Autodesk Inventor part; units mm, degrees
ref_plane "YZ Plane" through (0, 0, 0) normal (1, 0, 0) x (0, 1, 0)
ref_plane "XZ Plane" through (0, 0, 0) normal (0, 1, 0) x (-1, 0, 0)
ref_plane "XY Plane" through (0, 0, 0) normal (0, 0, 1) x (1, 0, 0)
sketch "Skizze1" plane through (0, 0, 0) normal (0, 0, 1) x (1, 0, 0)
  line L0 (0, 0) -> (10, 0)
  line L1 (10, 0) -> (10, 10)
  line L2 (10, 10) -> (0, 10)
  line L3 (0, 10) -> (0, 0)
  line L4 (70, 10) -> (80, 10)
  line L5 (80, 10) -> (80, 0)
  line L6 (80, 0) -> (70, 0)
  line L7 (70, 0) -> (70, 10)
  dimension "d0" = 10
  dimension "d1" = 10
  dimension "d2" = 10
  dimension "d3" = 10
  dimension "d4" = 60
extrude "Extrusion1" add sketch "Skizze1" along normal blind 7.5
sketch "Skizze2" plane through (0, 0, 7.5) normal (0, 0, 1) x (1, 0, 0)
  line L0 (80, 10) -> (70, 10)
  line L1 (70, 10) -> (70, 0)
  line L2 (70, 0) -> (80, 0)
  line L3 (80, 0) -> (80, 10)
  line L4 (0, 10) -> (80, 10)
  line L5 (80, 10) -> (80, 0)
  line L6 (80, 0) -> (0, 0)
  line L7 (0, 0) -> (0, 10)
extrude "Extrusion2" add sketch "Skizze2" along normal blind 4
fillet "Rundung1" radius 3 1 edges at (0, 5, 11.5)
fillet "Rundung1" radius 3 1 edges at (80, 5, 11.5)
fillet "Rundung1" radius 3 1 edges at (70, 5, 7.5)
fillet "Rundung1" radius 3 1 edges at (10, 5, 7.5)
sketch "Skizze3" plane through (0, 0, 7.5) normal (0, 0, -1) x (-1, 0, 0)
  line L0 (0, 0) -> (-50, 0)
  line L1 (-50, 0) -> (-50, 2)
  line L2 (-50, 2) -> (0, 2)
  line L3 (0, 2) -> (0, 0)
  dimension "d13" = 50
  dimension "d14" = 2
extrude "Extrusion3" add sketch "Skizze3" along normal blind 2
fillet "Rundung2" radius 1 1 edges at (50, 1, 5.5)
sketch "Skizze4" plane through (0, 0, 0) normal (0, 0, -1) x (-1, 0, 0)
  line L0 (0, 0) -> (-10, 0)
  line L1 (0, 10) -> (0, 0)
  circle A0 centre (-5, 5) radius 2.5
  dimension "d18" = 5
  dimension "d19" = 5
  dimension "d20" = 5
sketch "Skizze5" plane through (0, 0, 0) normal (0, 0, -1) x (-1, 0, 0)
  line L0 (-80, 0) -> (-70, 0)
  line L1 (-70, 0) -> (-70, 10)
  circle A0 centre (-75, 5) radius 2.5
  point P0 (0, 0)
  dimension "d21" = 5
  dimension "d22" = 5
  dimension "d23" = 5
extrude "Extrusion4" add sketch "Skizze4" along normal blind 3
extrude "Extrusion5" add sketch "Skizze5" along normal blind 3
properties part number "USB-Halter"
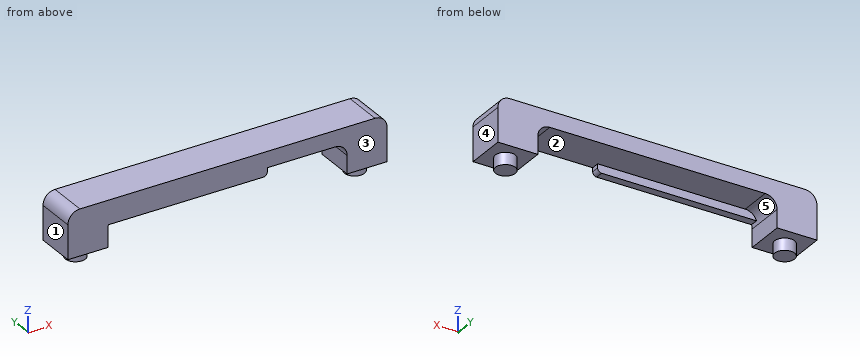
CAD build for the part. Positions are in the model's coordinates, mm. Face numbers are marked on the shaded views. A direction names the side the tool comes from. Give positions to 0.01 mm unless a question says otherwise; leave off trailing zeros. Loops run counter-clockwise (first coordinate to the right, second up) from the corner with the lowest first, then second, coordinate; pieces in that order, holes last. Notation, with made-up numbers: (15.5, 47) - (42.5, 47) arc R20 ccw to (42.5, 51) - close; hole circle Ø2 at (26.25, 8). An arc over 180 degrees is marked (long way). Put each result on its own line as item: value.
Q1. Slice it at C-C (y = 6). Give the cut face in (x, z).
Filled in:
outline: (0, 0) - (2.71, 0) - (2.71, -3) - (7.29, -3) - (7.29, 0) - (10, 0) - (10, 4.5) arc R3 cw to (13, 7.5) - (67, 7.5) arc R3 cw to (70, 4.5) - (70, 0) - (72.71, 0) - (72.71, -3) - (77.29, -3) - (77.29, 0) - (80, 0) - (80, 8.5) arc R3 ccw to (77, 11.5) - (3, 11.5) arc R3 ccw to (0, 8.5) - close
Q2. Mould opens along X. For the marked faces 1, 2 and 3 say: pulls with the +X half, pulls with the -X half, needs draft (parallel to the pull), parting line crosses it, or undercut.
Filled in:
face 1: pulls with the -X half
face 2: undercut
face 3: needs draft
Q3. Slice it at B-B (x = 75). Give the cut face in (y, z), plus the area to 3 significant figures.
Filled in:
outline: (0, 0) - (2.5, 0) - (2.5, -3) - (7.5, -3) - (7.5, 0) - (10, 0) - (10, 11.5) - (0, 11.5) - close
area: 130 mm²
Q4. Flat gauge pins, fed straight in: pin 1 (1.6 mm diameter, centred on x = 38, y = 0.5, fed in from -Z); pin 2 (2 mm diameter, centred on x = 37.5, z = 6, fed in from +Y). Where does each tip first touch, or does it go through?
Filled in:
pin 1: stops at z = 5.5
pin 2: stops at y = 2
Q5. Probe line 1 along X through (y, z) = (2.25, 4.75); line 2 along Z through (x, y) = (39, 1.25); line 3 along X through (y, z) = (4, 5.75). List the from-to ranges inside material, lowest first.
Filled in:
line 1: x = 0 to 10.01, 69.99 to 80
line 2: z = 5.5 to 11.5
line 3: x = 0 to 10.27, 69.73 to 80
Q6. Slice it at A-A (z = 3.75). Give the cut face in (x, y), plus the area to 3 significant figures.
Filled in:
outline: (0, 0) - (10, 0) - (10, 10) - (0, 10) - close; (70, 0) - (80, 0) - (80, 10) - (70, 10) - close
area: 200 mm²
Q7. Slice it at D-D (x = 19). Give the cut face in (y, z).
Filled in:
outline: (0, 5.5) - (2, 5.5) - (2, 7.5) - (10, 7.5) - (10, 11.5) - (0, 11.5) - close
Q8. Tool access for the marked faces 4 and 5: list every direction of +Z, -Z, +X, -X, +Y, -Y with a clear straight run to the whole face (end or side of a thin tool).
Filled in:
face 4: +Z, -Z, +X, +Y, -Y
face 5: -Z, +Y
